Geometry check sheet. Reference: the model listing, model coordinates, mm. A direction names the side the tool comes from. Round coordinates to 2 decimals unless told otherwise and drop trailing zeros. Order: outer loops, then holes, each group sorted by start corner. A loop starts at its lowest first (then second) coordinate and runs counter-clockwise, first axis right, second up. Notation, with made-up numbers: (6, -27) -> (50, -27) arc R13 cw to (50, -6) -> close; hole circle Ø9 at (-10.5, 24). An arc over 180 degrees is marked (long way). Use a Markdown table: item, result. Add a question column.
Item 1: Material ranges on probe 1 along X at (y, z) = (3.7, 0) (3 decimals); probe 2 along X at (y, z) = (0.5, -0.5); probe 3 along Y at (x, z) = (0, 2.75), recorded low to high. Write a range as [from, to].
Item 2: Gauge pin test, flat ends, axial feed: pin 1 Ø4 at (y, z) = (-1.5, -0.5) entering from +X; pin 2 Ø4 at (x, z) = (0.5, 1) entering from -Y; pin 3 Ø2.5 at (x, z) = (4, 0) entering from -Y. Record the tip position at first contact, or that the pin passes through.
Item 3: Sectioned sample at B-B, the plane y = 2.25. Record the cut outline in (x, z) (3 decimals), and give its area (3 significant figures).
Item 4: Mould release check, pull along Z, two halves, no side actions. Record for faces 3 (the cylindrical face through (6.156, 2.535, -0.283)), 4 (the flat face through (15.7, 4.5, 0)), 5 (the cylindrical face through (-10.315, 2.535, -0.228)), 6 (the conical face through (-26, 4.6, 3.98)): pulls with the +Z half, pulls with the -Z half, needs draft (parallel to the pull), parting line crosses it, or undercut.
Item 5: Set-up check for faces 1 (the cylindrical face through (-26.62, -1.08, -1.34)), 2 (the flat face through (-5.1, 0.5, 4.5)): record each of +Z, -Z, +X, -X, +Y, -Y from which the full face is reachable in a straight line by a thin tool's end or side.
Item 6: Sectioned sample at A-A, the plane x = 11.95. Record the cut outline in (y, z).
Item 7: Sectioned sample at D-D, the plane x = -1.5. Record the cut outline in (y, z), and give its area (3 significant figures).
Item 8: Sectioned sample at C-C, the plane z = 0. Record the cut outline in (x, y) (3 decimals).
from build123d import *

# Parameters (mm, degrees)
SKETCH1_W           = 54
SKETCH1_H           = 10
BOSS_EXTRUDE1_DEPTH = 5
SKETCH3_R           = 1.5
SKETCH3_R_2         = 2.175
SKETCH3_R_3         = 1.75
CUT_EXTRUDE1_DEPTH  = 7
FILLET1_R           = 2
SKETCH4_R           = 2.9
SKETCH4_R_2         = 1.5
BOSS_EXTRUDE2_DEPTH = 2.5
SKETCH5_W           = 14.628032649
SKETCH5_H           = 11.072623212
CUT_EXTRUDE2_DEPTH  = 10
FILLET2_R           = 2
CHAMFER1_SIZE       = 1


with BuildPart() as part:
    # Sketch1 → Boss-Extrude1 (new body)
    with BuildSketch(Plane(origin=(0, 0, 0), x_dir=(1, 0, 0), z_dir=(0, 1, 0))):
        Rectangle(SKETCH1_W, SKETCH1_H)
    extrude(amount=BOSS_EXTRUDE1_DEPTH)

    # Sketch3 → Cut-Extrude1 (cut)
    with BuildSketch(Plane(origin=(0, 5, 0), x_dir=(1, 0, 0), z_dir=(0, 1, 0))):
        with Locations(Location((-24.05, 0, 0), (0, 0, 270))):
            Circle(SKETCH3_R)
        with Locations(Location((4, 0, 0), (0, 0, 270))):
            Circle(SKETCH3_R_2)
        with Locations(Location((-12.05, 0, 0), (0, 0, 270))):
            Circle(SKETCH3_R_3)
        with Locations(Location((11.95, 0, 0), (0, 0, 270))):
            Circle(SKETCH3_R_3)
    extrude(amount=-CUT_EXTRUDE1_DEPTH, mode=Mode.SUBTRACT)

    # Fillet1
    fillet1_edges = [part.edges().sort_by_distance(p)[0] for p in [
        (27, 2.5, 5),
        (-27, 2.5, 5),
        (-27, 2.5, -5),
        (27, 2.5, -5),
    ]]
    fillet(fillet1_edges, radius=FILLET1_R)

    # Sketch4 → Boss-Extrude2 (add)
    with BuildSketch(Plane.XZ):
        with Locations(Location((-24.05, 0, 0), (0, 0, 270))):
            Circle(SKETCH4_R)
        with Locations(Location((-24.05, 0, 0), (0, 0, 90))):
            Circle(SKETCH4_R_2, mode=Mode.SUBTRACT)
    extrude(amount=BOSS_EXTRUDE2_DEPTH)

    # Sketch5 → Cut-Extrude2 (cut)
    with BuildSketch(Plane(origin=(0, 5, 0), x_dir=(1, 0, 0), z_dir=(0, 1, 0))):
        with Locations((23.514016324, -0.536311606)):
            Rectangle(SKETCH5_W, SKETCH5_H)
    extrude(amount=-CUT_EXTRUDE2_DEPTH, mode=Mode.SUBTRACT)

    # Fillet2
    fillet2_edges = [part.edges().sort_by_distance(p)[0] for p in [
        (16.2, 2.5, 5),
        (16.2, 2.5, -5),
    ]]
    fillet(fillet2_edges, radius=FILLET2_R)

    # Chamfer1
    # the kernel refuses this chamfer: 1 mm, written as the material it takes off along each edge
    with BuildSketch(Plane(origin=(14.2, 0, -3), x_dir=(0, 0, -1), z_dir=(-1, 0, 0))) as chamfer1_piece_1:
        Polygon((2 - CHAMFER1_SIZE, 0), (2, -CHAMFER1_SIZE), (2, 0), align=None)
    revolve(axis=Axis((14.2, 0, -3), (0, -1, 0)), revolution_arc=90, mode=Mode.SUBTRACT)
    with BuildSketch(Plane(origin=(14.2, 0, 5), x_dir=(0, -0.027495876610586365, -0.9996219169112968), z_dir=(-1, 0, 0)), Plane(origin=(-25, 5, -5), x_dir=(0, -0.9996219169112968, -0.027495876610586487), z_dir=(1, 0, 0))) as chamfer1_piece_2:
        Polygon((CHAMFER1_SIZE * 0.999621916911, -CHAMFER1_SIZE * 0.0274958766106), (-CHAMFER1_SIZE * 0.0274958766106, -CHAMFER1_SIZE * 0.999621916911), (0, 0), align=None)
    extrude(amount=39.2, mode=Mode.SUBTRACT)
    with BuildSketch(Plane(origin=(-27, 0, 3), x_dir=(0.9996219169112968, -0.02749587661058639, 0), z_dir=(0, 0, -1))) as chamfer1_piece_3_section:
        Polygon((CHAMFER1_SIZE * 0.999621916911, -CHAMFER1_SIZE * 0.0274958766106), (-CHAMFER1_SIZE * 0.0274958766106, -CHAMFER1_SIZE * 0.999621916911), (0, 0), align=None)
    chamfer1_piece_3 = extrude(amount=6, mode=Mode.PRIVATE)
    chamfer1_piece_3 = chamfer1_piece_3 - Plane(origin=(-24.05, 0.490897833, 0), x_dir=(0, 0, -1), z_dir=(0, 1, 0)) * Cylinder(2.9, 16, mode=Mode.PRIVATE)
    add(chamfer1_piece_3, mode=Mode.SUBTRACT)
    with BuildSketch(Plane(origin=(-25, 0, 3), x_dir=(-1, 0, 0), z_dir=(0, 0, -1))) as chamfer1_piece_4:
        Polygon((2 - CHAMFER1_SIZE, 0), (2, CHAMFER1_SIZE), (2, 0), align=None)
    revolve(axis=Axis((-25, 0, 3), (0, 1, 0)), revolution_arc=90, mode=Mode.SUBTRACT)
    with BuildSketch(Plane(origin=(-25, 0, -3), x_dir=(0, 0, -1), z_dir=(1, 0, 0))) as chamfer1_piece_5:
        Polygon((2 - CHAMFER1_SIZE, 0), (2, CHAMFER1_SIZE), (2, 0), align=None)
    revolve(axis=Axis((-25, 0, -3), (0, 1, 0)), revolution_arc=90, mode=Mode.SUBTRACT)
    with BuildSketch(Plane(origin=(-27, 5, 3), x_dir=(0.9996219169112968, 0.02749587661058651, 0), z_dir=(0, 0, -1))) as chamfer1_piece_6:
        Polygon((CHAMFER1_SIZE * 0.999621916911, CHAMFER1_SIZE * 0.0274958766106), (-CHAMFER1_SIZE * 0.0274958766106, CHAMFER1_SIZE * 0.999621916911), (0, 0), align=None)
    extrude(amount=6, mode=Mode.SUBTRACT)
    with BuildSketch(Plane(origin=(14.2, 5, 5), x_dir=(0, 0.027495876610586487, -0.9996219169112968), z_dir=(-1, 0, 0)), Plane(origin=(-25, 0, -5), x_dir=(0, 0.9996219169112968, -0.027495876610586494), z_dir=(1, 0, 0))) as chamfer1_piece_7:
        Polygon((CHAMFER1_SIZE * 0.999621916911, CHAMFER1_SIZE * 0.0274958766106), (-CHAMFER1_SIZE * 0.0274958766106, CHAMFER1_SIZE * 0.999621916911), (0, 0), align=None)
    extrude(amount=39.2, mode=Mode.SUBTRACT)
    with BuildSketch(Plane(origin=(-25, 5, 3), x_dir=(-1, 0, 0), z_dir=(0, 0, -1))) as chamfer1_piece_8:
        Polygon((2 - CHAMFER1_SIZE, 0), (2, -CHAMFER1_SIZE), (2, 0), align=None)
    revolve(axis=Axis((-25, 5, 3), (0, 1, 0)), revolution_arc=90, mode=Mode.SUBTRACT)
    with BuildSketch(Plane(origin=(-25, 5, -3), x_dir=(0, 0, -1), z_dir=(1, 0, 0))) as chamfer1_piece_9:
        Polygon((2, -CHAMFER1_SIZE), (2 - CHAMFER1_SIZE, 0), (2, 0), align=None)
    revolve(axis=Axis((-25, 5, -3), (0, 1, 0)), revolution_arc=90, mode=Mode.SUBTRACT)
    with BuildSketch(Plane(origin=(16.2, 0, -3), x_dir=(-0.9996219169112968, -0.02749587661058639, 0), z_dir=(0, 0, 1)), Plane(origin=(16.2, 5, 3), x_dir=(-0.9996219169112968, 0.02749587661058651, 0), z_dir=(0, 0, -1))) as chamfer1_piece_10:
        Polygon((CHAMFER1_SIZE * 0.999621916911, -CHAMFER1_SIZE * 0.0274958766106), (-CHAMFER1_SIZE * 0.0274958766106, -CHAMFER1_SIZE * 0.999621916911), (0, 0), align=None)
    extrude(amount=6, mode=Mode.SUBTRACT)
    with BuildSketch(Plane(origin=(14.2, 5, 3), x_dir=(1, 0, 0), z_dir=(0, 0, -1))) as chamfer1_piece_11:
        Polygon((2 - CHAMFER1_SIZE, 0), (2, CHAMFER1_SIZE), (2, 0), align=None)
    revolve(axis=Axis((14.2, 5, 3), (0, -1, 0)), revolution_arc=90, mode=Mode.SUBTRACT)
    with BuildSketch(Plane(origin=(14.2, 5, -3), x_dir=(0, 0, -1), z_dir=(-1, 0, 0))) as chamfer1_piece_12:
        Polygon((2, CHAMFER1_SIZE), (2 - CHAMFER1_SIZE, 0), (2, 0), align=None)
    revolve(axis=Axis((14.2, 5, -3), (0, -1, 0)), revolution_arc=90, mode=Mode.SUBTRACT)
    with BuildSketch(Plane(origin=(14.2, 0, 3), x_dir=(1, 0, 0), z_dir=(0, 0, -1))) as chamfer1_piece_13:
        Polygon((2 - CHAMFER1_SIZE, 0), (2, -CHAMFER1_SIZE), (2, 0), align=None)
    revolve(axis=Axis((14.2, 0, 3), (0, -1, 0)), revolution_arc=90, mode=Mode.SUBTRACT)


solid = part.part
Found:
| question | item | result |
|---|---|---|
| 1 | probe 1 | x = [-27, -25.55], [-22.55, -13.8], [-10.3, 1.825], [6.175, 10.2], [13.7, 16.2] |
| 1 | probe 2 | x = [-26.91, -25.46], [-22.64, -13.73], [-10.37, 1.88], [6.12, 10.27], [13.63, 15.7] |
| 1 | probe 3 | y = [0, 5] |
| 2 | pin 1 | stops at x = 15.7 |
| 2 | pin 2 | stops at y = 0 |
| 2 | pin 3 | passes through |
| 3 | outline | (-27, -3) arc R2 ccw to (-25, -5) -> (14.2, -5) arc R2 ccw to (16.2, -3) -> (16.2, 3) arc R2 ccw to (14.2, 5) -> (-25, 5) arc R2 ccw to (-27, 3) -> close; hole circle Ø3 at (-24.05, 0); hole circle Ø3.5 at (-12.05, 0); hole circle Ø4.35 at (4, 0); hole circle Ø3.5 at (11.95, 0) |
| 3 | area | 387 mm2 |
| 4 | face 3 | undercut |
| 4 | face 4 | needs draft |
| 4 | face 5 | undercut |
| 4 | face 6 | pulls with the +Z half |
| 5 | face 1 | -Y |
| 5 | face 2 | +Z, +X, -X, -Y |
| 6 | outline | (0, -4) -> (1, -5) -> (4, -5) -> (5, -4) -> (5, -1.75) -> (0, -1.75) -> close; (0, 1.75) -> (5, 1.75) -> (5, 4) -> (4, 5) -> (1, 5) -> (0, 4) -> close |
| 7 | outline | (0, -4) -> (1, -5) -> (4, -5) -> (5, -4) -> (5, 4) -> (4, 5) -> (1, 5) -> (0, 4) -> close |
| 7 | area | 48.0 mm2 |
| 8 | outline | (-27, 1) -> (-26.95, 0.95) -> (-26.95, -2.5) -> (-25.55, -2.5) -> (-25.55, 5) -> (-26, 5) -> (-27, 4) -> close; (-22.55, -2.5) -> (-21.15, -2.5) -> (-21.15, 0) -> (-13.8, 0) -> (-13.8, 5) -> (-22.55, 5) -> close; (-10.3, 0) -> (1.825, 0) -> (1.825, 5) -> (-10.3, 5) -> close; (6.175, 0) -> (10.2, 0) -> (10.2, 5) -> (6.175, 5) -> close; (13.7, 0) -> (15.2, 0) -> (16.2, 1) -> (16.2, 4) -> (15.2, 5) -> (13.7, 5) -> close |
